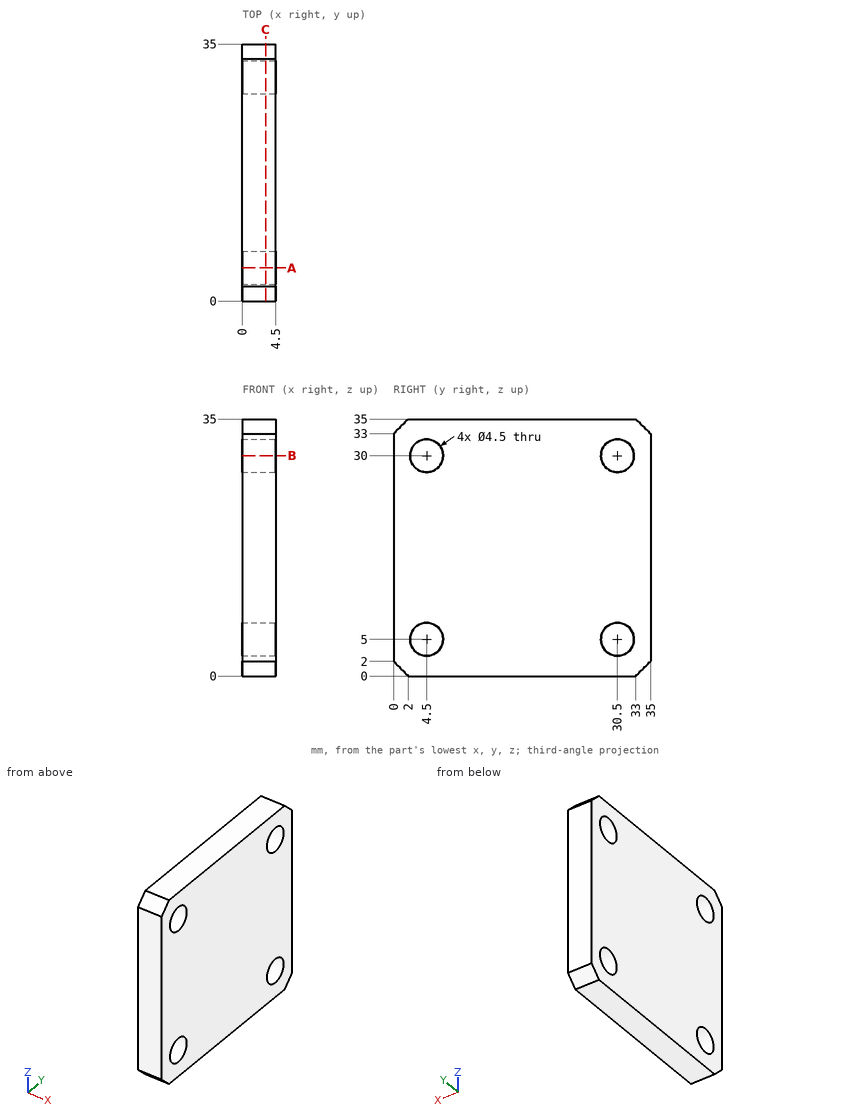
Study the drawing (mm; zero at the part's minimum x, y, z) and answer. Give positions to 0.01 mm unless a question says otherwise; leave off trailing zeros. Write each loop counter-clockwise with the first axis right and the second up, starting at its lowest first coordinate (ties: lowest second). Pieces come first, ordered by that corner, then holes. Notation, with made-up numbers: (-14, 87.5) - (-3, 87.5) arc R22 ccw to (-3, 118.5) - close; hole circle Ø6 at (23.25, 29). An arc over 180 degrees is marked (long way). Use a Markdown table: item, result.
1. This flat-tipped pin is pushed along its axis until it touches: P1, Ø6, axis at y = 19.5, z = 21, coming from the -X side. Where does it stop, or does it pass through?
Values follow:
| item | result |
|---|---|
| P1 | stops at x = 0 |
2. Find the intervals of material crossed by probe 1 along Y at (x, z) = (1.8, 30); probe 2 along Z at (x, y) = (1.75, 30.5); probe 3 along Y at (x, z) = (1.8, 31), in increasing order. Write a range as from..to.
Values follow:
| item | result |
|---|---|
| probe 1 | y = 0..2.25, 6.75..28.25, 32.75..35 |
| probe 2 | z = 0..2.75, 7.25..27.75, 32.25..35 |
| probe 3 | y = 0..2.48, 6.52..28.48, 32.52..35 |
3. Section B-B on z = 30 is taken. Write down the section's boundary in (x, y).
Values follow:
| item | result |
|---|---|
| outline | (0, 0) - (4.5, 0) - (4.5, 2.25) - (0, 2.25) - close; (0, 6.75) - (4.5, 6.75) - (4.5, 28.25) - (0, 28.25) - close; (0, 32.75) - (4.5, 32.75) - (4.5, 35) - (0, 35) - close |
4. Section C-C on x = 3.15 is taken. Write down the section's boundary in (y, z), plus the area to 3 significant figures.
Values follow:
| item | result |
|---|---|
| outline | (0, 2) - (2, 0) - (33, 0) - (35, 2) - (35, 33) - (33, 35) - (2, 35) - (0, 33) - close; hole circle Ø4.5 at (4.5, 5); hole circle Ø4.5 at (4.5, 30); hole circle Ø4.5 at (30.5, 5); hole circle Ø4.5 at (30.5, 30) |
| area | 1,150 mm² |
5. Section A-A on y = 4.5 is taken. Write down the section's boundary in (x, z), plus the area to 3 significant figures.
Values follow:
| item | result |
|---|---|
| outline | (0, 0) - (4.5, 0) - (4.5, 2.75) - (0, 2.75) - close; (0, 7.25) - (4.5, 7.25) - (4.5, 27.75) - (0, 27.75) - close; (0, 32.25) - (4.5, 32.25) - (4.5, 35) - (0, 35) - close |
| area | 117 mm² |
